Design review of the part shown in the three views and the two pictorial views. Dimensions are in mm from the part's minimum x, y and z. Coordinates: 2 decimals unless noted, no trailing zeros. Write each loop counter-clockwise with the first axis right and the second up, starting at its lowest first coordinate (ties: lowest second). Pieces come first, ordered by that corner, then holes. Notation, with made-up numbers: (-31, 39) - (5, 39) arc R28 ccw to (5, 57) - close; hole circle Ø11 at (89, 32.25). An arc over 180 degrees is marked (long way). Write each question's results on one line, items separated by ' | '.
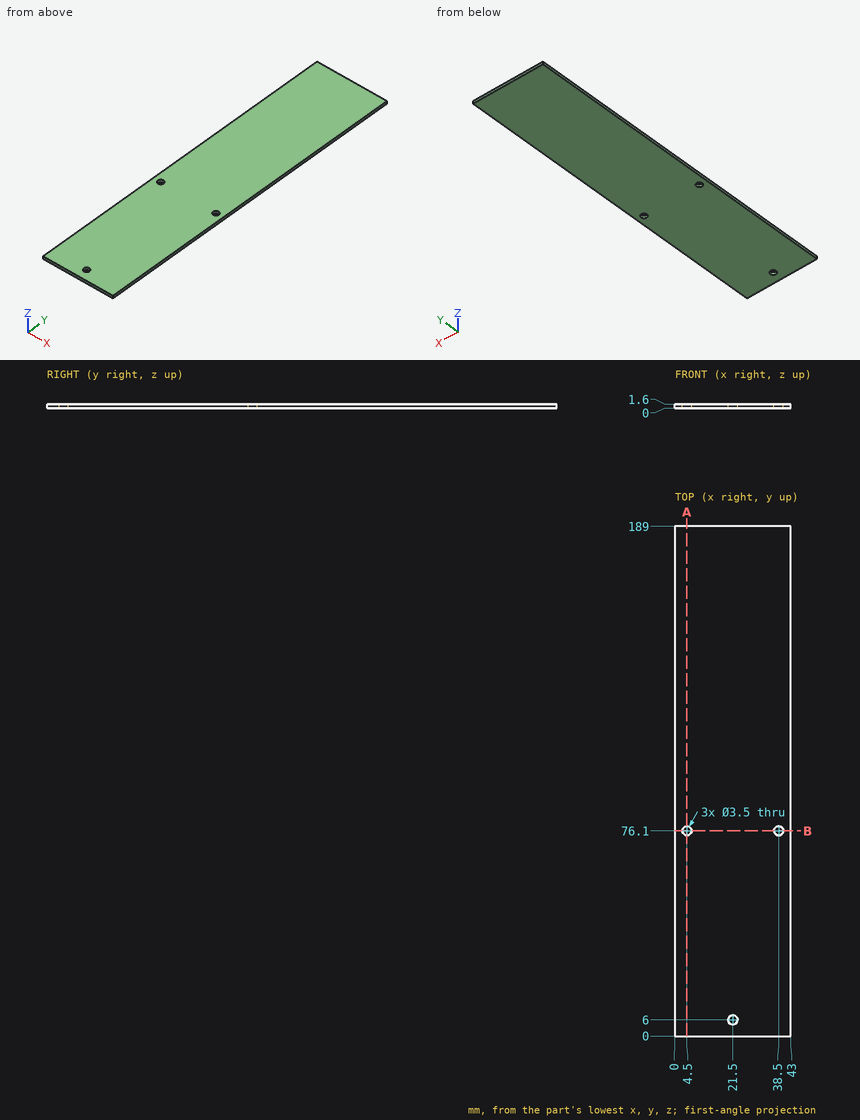
Q1. Take a section at B-B on y = 76.1. State the section outline as (x, z) points.
Results found:
outline: (0, 0) - (2.75, 0) - (2.75, 1.6) - (0, 1.6) - close; (6.25, 0) - (36.75, 0) - (36.75, 1.6) - (6.25, 1.6) - close; (40.25, 0) - (43, 0) - (43, 1.6) - (40.25, 1.6) - close
Q2. For pin 1 (2 mm diameter, centred on x = 4.5, y = 76.1, fed in from -Z), flat-tipped, find the tip position at first contact; note if it passes through.
Results found:
pin 1: through
Q3. Take a section at A-A on x = 4.5. State the section outline as (y, z) points.
Results found:
outline: (0, 0) - (74.35, 0) - (74.35, 1.6) - (0, 1.6) - close; (77.85, 0) - (189, 0) - (189, 1.6) - (77.85, 1.6) - close
Q4. Wall thickness on line 1 along X through (y, z) = (76.1, 0.4); line 2 along Y through (x, z) = (21.5, 0.6); line 3 along X through (y, z) = (6, 1.25): over which ranges is each line inside the solid? List them lowest first. Write a range as from..to.
Results found:
line 1: 0..2.75, 6.25..36.75, 40.25..43 | line 2: 0..4.25, 7.75..189 | line 3: 0..19.75, 23.25..43
